Answer from the drawing. Dimensions are ordinates in mm from the lowest x, y and z of the part. A direction names the side the tool comes from. Coordinates: 2 decimals unless noted, no trailing zeros. Loops run counter-clockwise (first coordinate to the right, second up) from the corner with the lowest first, then second, coordinate; pieces in that order, holes last. Notation, with made-up numbers: M 25.5,-10 L 45.5,-10 A15 ccw 45.5,17 Z; hole C 57,27.25 d1. An arc over 180 degrees is marked long. Answer as CSV lines item,"result". Start each with the question number.
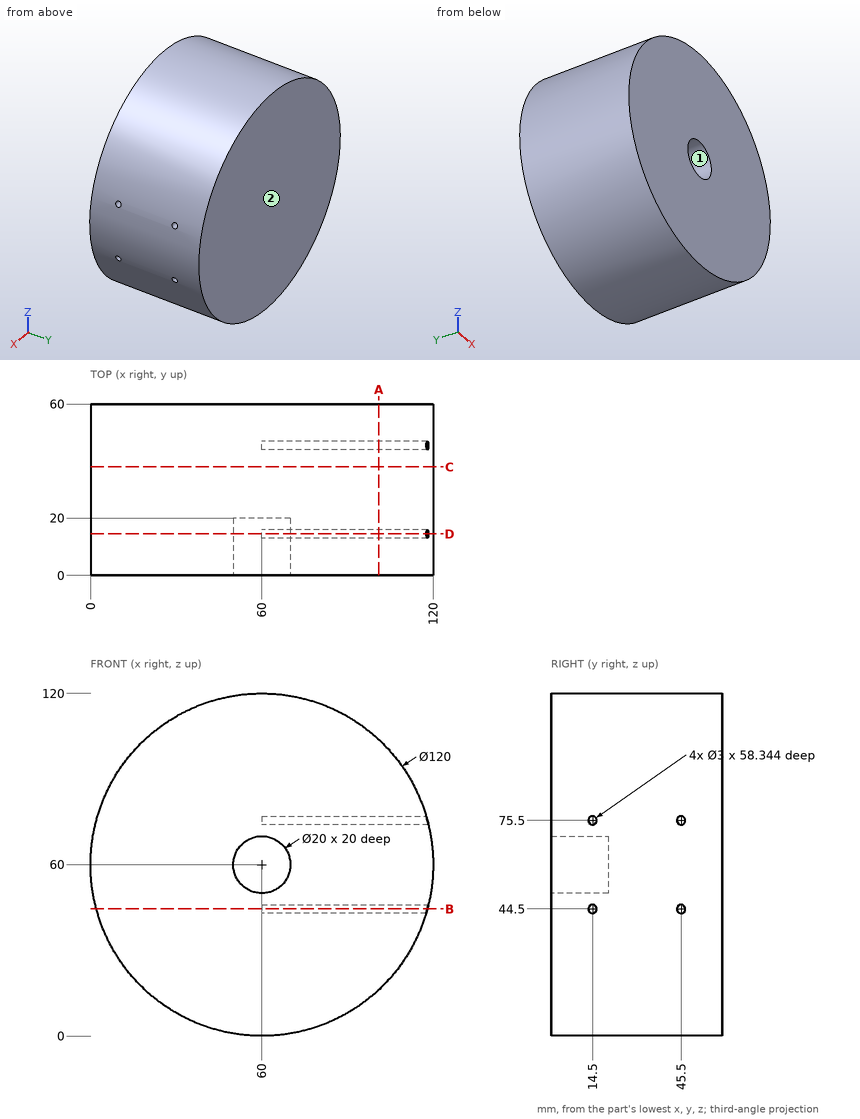
Item 1: Section A-A on x = 101 is taken. Determine the outline of the cut face in (y, z).
Item 2: Each of these flat-tipped pins is pushed along its axis until it touches: P1, Ø1, axis at x = 52.5, y = 48, coming from the -Z side; P2, Ø1.5, axis at x = 70.5, y = 40.5, coming from the -Z side; P3, Ø1.5, axis at y = 11, z = 22.5, coming from the -X side. Where does it stop, or does it pass through?
Item 3: Section B-B on z = 44.5 is taken. Determine the outline of the cut face in (x, y).
Item 4: Consider line 1 (Y direction, x = 87, z = 44.5); line 2 (Z direction, x = 79, y = 14); line 3 (X direction, y = 11, z = 60). Determine where each line is inside the solid, lowest interval first.
Item 5: Section C-C on y = 38 is taken. Determine the outline of the cut face in (x, z), then the cut area to 3 significant figures.
Item 6: Section D-D on y = 14.5 is taken. Determine the outline of the cut face in (x, z), then the cut area to 3 significant figures.
Item 7: For the marked faces 1 and 2, determine the directions among +Z, -Z, +X, -X, +Y, -Y from which every point of the face is accessible in a straight line to the end or side of a thin tool.
Results are:
1,outline,"M 0,16.19 L 60,16.19 L 60,103.81 L 0,103.81 Z; hole C 14.5,44.5 d3; hole C 14.5,75.5 d3; hole C 45.5,44.5 d3; hole C 45.5,75.5 d3"
2,P1,"z = 0.41"
2,P2,"z = 0.8"
2,P3,"x = 12.57"
3,outline,"M 2.04,0 L 117.96,0 L 117.96,13 L 60,13 L 60,16 L 117.96,16 L 117.96,44 L 60,44 L 60,47 L 117.96,47 L 117.96,60 L 2.04,60 Z"
4,line 1,"0 to 13, 16 to 44, 47 to 60"
4,line 2,"3.09 to 43.09, 45.91 to 74.09, 76.91 to 116.91"
4,line 3,"0 to 50, 70 to 120"
5,outline,"C 60,60 d120"
5,area,"11,300 mm²"
6,outline,"M 60,43 L 60,46 L 118.34,46 A60 ccw 118.34,74 L 60,74 L 60,77 L 117.54,77 A60 ccw long 117.54,43 Z; hole C 60,60 d20"
6,area,"10,600 mm²"
7,face 1,"-Y"
7,face 2,"+Z, -Z, +X, -X, +Y"
